Can you work these out from the model? Positions are in its coordinate system, mm. A direction names the side the tool comes from. Coordinates: 2 decimals unless noted, no trailing zeros. Loops run counter-clockwise (first coordinate to the right, second up) from the corner with the lowest first, then second, coordinate; pieces in that order, holes last. Notation, with made-up numbers: (-32.75, -2) -> (-1.75, -2) arc R19 ccw to (-1.75, 17) -> close; hole circle Ø5 at (62.25, 0). An arc over 180 degrees is marked (long way). Use one line per item in the form item = value. Start each with the question number.
(1) I need wall thicknesses on line 1 (Y direction, x = -33.75, z = 2.5); line 2 (X direction, y = 0.5, z = 0.5); line 3 (X direction, y = 18, z = 1.75). Which ranges of each line are inside material? Lowest first, please. Write a range as [from, to].
(2) I'm going to push a flat-ended pin straight in: pin 1 (3 mm diameter, centred on x = -33, z = 4.5, fed in from +Y). Where does the tip first touch, or does it pass through?
(3) Thinking about a two-plate mould opening in X: for faces 4 (the cylindrical face through (-28.755, 0.22, 4.93)), 5 (the flat face through (-1, 0, 10)), 6 (the flat face through (25, 0, 5)), 7 (the flat face through (-25, -16, 5)), which applies, released by +X, released by -X, zero draft, split by the parting line, or undercut?
(4) Imagine slicing it at B-B (y = 0). List the corners of the cut face in (x, z) for me, plus the area to 3 significant figures.
(5) Imagine slicing it at D-D (y = 11). List the corners of the cut face in (x, z) for me.
(6) On a 3-axis mill with a long thin cutter (end or side, diameter ignored), from which of +Z, -Z, +X, -X, +Y, -Y can I reach the whole of each face in a straight line? I mean faces 1 (the flat face through (-32, 6.25, 5)), 2 (the flat face through (-32, -6.25, 5)), 3 (the flat face through (0, 25, 5)). Say none if no direction works.
(7) Imagine slicing it at A-A (x = -33.75). List the corners of the cut face in (y, z) for me, plus the area to 3 significant figures.
(8) Imagine slicing it at C-C (z = 1.75). List the corners of the cut face in (x, y) for me.
```python
from build123d import *

# Parameters (mm, degrees)
SKETCH1_W           = 50
SKETCH1_H           = 50
BOSS_EXTRUDE1_DEPTH = 10
SKETCH6_W           = 10
SKETCH6_H           = 12.5
BOSS_EXTRUDE5_DEPTH = 15
SKETCH7_R           = 5
CUT_EXTRUDE2_DEPTH  = 49.218253805


with BuildPart() as part:
    # Sketch1 → Boss-Extrude1 (new body)
    with BuildSketch(Plane.XY):
        Rectangle(SKETCH1_W, SKETCH1_H)
    extrude(amount=BOSS_EXTRUDE1_DEPTH)

    # Sketch6 → Boss-Extrude5 (add)
    with BuildSketch(Plane.ZY.offset(25)):
        with Locations((5, 0)):
            Rectangle(SKETCH6_W, SKETCH6_H)
    extrude(amount=BOSS_EXTRUDE5_DEPTH)

    # Sketch7 → Cut-Extrude2 (cut, through all)
    with BuildSketch(Plane(origin=(0, 0, 0), x_dir=(-1, 0, 0), z_dir=(0, 0, -1))):
        with Locations((33.75, 0)):
            Circle(SKETCH7_R)
    extrude(amount=-CUT_EXTRUDE2_DEPTH, mode=Mode.SUBTRACT)


solid = part.part
```
Worked out:
q1.line_1 = [-6.25, -5], [5, 6.25]
q1.line_2 = [-40, -38.72], [-28.78, 25]
q1.line_3 = [-25, 25]
q2.pin_1 = 6.25
q3.face_4 = undercut
q3.face_5 = zero draft
q3.face_6 = released by +X
q3.face_7 = released by -X
q4.outline = (-40, 0) -> (-38.75, 0) -> (-38.75, 10) -> (-40, 10) -> close; (-28.75, 0) -> (25, 0) -> (25, 10) -> (-28.75, 10) -> close
q4.area = 550 mm2
q5.outline = (-25, 0) -> (25, 0) -> (25, 10) -> (-25, 10) -> close
q6.face_1 = +Z, -Z, -X, +Y
q6.face_2 = +Z, -Z, -X, -Y
q6.face_3 = +Z, -Z, +X, -X, +Y
q7.outline = (-6.25, 0) -> (-5, 0) -> (-5, 10) -> (-6.25, 10) -> close; (5, 0) -> (6.25, 0) -> (6.25, 10) -> (5, 10) -> close
q7.area = 25.0 mm2
q8.outline = (-40, -6.25) -> (-25, -6.25) -> (-25, -25) -> (25, -25) -> (25, 25) -> (-25, 25) -> (-25, 6.25) -> (-40, 6.25) -> close; hole circle Ø10 at (-33.75, 0)
